Input: part model. Units: mm. Frame: model coordinates. A direction names the side the tool comes from. Coordinates: 2 decimals unless noted, no trailing zeros. Loops run counter-clockwise (first coordinate to the right, second up) from the corner with the lowest first, then second, coordinate; pieces in that order, holes last. Notation, with made-up numbers: (52, 70.25) - (83, 70.25) arc R23 cw to (83, 80.25) - close; hole circle Ø4 at (46, -33.75). An arc over 180 degrees is marked (long way). Answer as CSV lines item,"result". Start each with the question number.
```python
from build123d import *

# Parameters (mm, degrees)
SKETCH1_R           = 4.25
BOSS_EXTRUDE1_DEPTH = 4
SKETCH2_W           = 11.313708498
SKETCH2_H           = 11.313708498
BOSS_EXTRUDE2_DEPTH = 2
SKETCH3_R           = 4.1
CUT_EXTRUDE1_DEPTH  = 2


with BuildPart() as part:
    # Sketch1 → Boss-Extrude1 (new body)
    with BuildSketch(Plane(origin=(0, 0, 0), x_dir=(1, 0, 0), z_dir=(0, 1, 0))):
        with Locations(Location((0, 0, 0), (0, 0, 270))):
            Circle(SKETCH1_R)
    extrude(amount=BOSS_EXTRUDE1_DEPTH)

    # Sketch2 → Boss-Extrude2 (add)
    with BuildSketch(Plane(origin=(0, 4, 0), x_dir=(1, 0, 0), z_dir=(0, 1, 0))):
        Rectangle(SKETCH2_W, SKETCH2_H)
    extrude(amount=BOSS_EXTRUDE2_DEPTH)

    # Sketch3 → Cut-Extrude1 (cut)
    with BuildSketch(Plane.XZ):
        with Locations(Location((0, 0, 0), (0, 0, 270))):
            Circle(SKETCH3_R)
    extrude(amount=-CUT_EXTRUDE1_DEPTH, mode=Mode.SUBTRACT)


solid = part.part
```
Item 1: Material intervals for probe 1 along Y at (x, z) = (-1, 1.75); probe 2 along Y at (x, z) = (0, 4.5); probe 3 along Z at (x, y) = (2, 0.95), sorted ascending.
Item 2: Section query C-C, the plane z = -2.75. Output: boundary loops of the cut face in (x, y), and give its area (3 significant figures).
Item 3: Section query A-A, the plane x = 0. Output: boundary loops of the cut face in (y, z), and give its area (3 significant figures).
Item 4: Section query D-D, the plane z = 4.5. Output: boundary loops of the cut face in (x, y).
Item 5: Section query B-B, the plane y = 1.8. Output: boundary loops of the cut face in (x, z), and give its area (3 significant figures).
Item 6: Set-up query: faces 5 (the flat face through (-5.657, 5, 0)), 6 (the flat face through (2, 4, -4)). Return all of +Z, -Z, +X, -X, +Y, -Y with unobstructed straight access to the full face (end or side cutting, diameter ignored); none if empty.
Item 7: Draft query along Z for faces 1 (the flat face through (5.657, 5, 0)), 2 (the cylindrical face through (4.214, 1.972, -0.553)), 3 (the flat face through (0, 2, 0)), 4 (the cylindrical face through (4.065, 0.986, 0.534)). Return one class per face: pulls with the +Z half, pulls with the -Z half, needs draft (parallel to the pull), parting line crosses it, or undercut.
Item 8: Contact query for flat-ended pins moving along their axis: P1, Ø4, axis at x = 1.5, z = 0, coming from the -Y side; P2, Ø3, axis at x = 3.5, z = 1.5, coming from the -Y side; P3, Ø1, axis at x = 2, y = 1.5, coming from the -Z side. Output: stop coordinate, or through.
Response values:
1,probe 1,"y = 2 to 6"
1,probe 2,"y = 4 to 6"
1,probe 3,"z = -3.75 to -3.58, 3.58 to 3.75"
2,outline,"(-5.66, 4) - (-3.24, 4) - (-3.24, 0) - (-3.04, 0) - (-3.04, 2) - (3.04, 2) - (3.04, 0) - (3.24, 0) - (3.24, 4) - (5.66, 4) - (5.66, 6) - (-5.66, 6) - close"
2,area,"36.4 mm²"
3,outline,"(0, -4.25) - (4, -4.25) - (4, -5.66) - (6, -5.66) - (6, 5.66) - (4, 5.66) - (4, 4.25) - (0, 4.25) - (0, 4.1) - (2, 4.1) - (2, -4.1) - (0, -4.1) - close"
3,area,"40.2 mm²"
4,outline,"(-5.66, 4) - (5.66, 4) - (5.66, 6) - (-5.66, 6) - close"
5,outline,"circle Ø8.5 at (0, 0); hole circle Ø8.2 at (0, 0)"
5,area,"3.93 mm²"
6,face 5,"+Z, -Z, -X, +Y, -Y"
6,face 6,"-Y"
7,face 1,"needs draft"
7,face 2,"parting line crosses it"
7,face 3,"undercut"
7,face 4,"undercut"
8,P1,"stops at y = 2"
8,P2,"stops at y = 0"
8,P3,"stops at z = -3.98"
